from build123d import *

# Parameters (mm, degrees)
F4_DEPTH        = 101.6027760721
F5_R            = 1.5875
F6_DEPTH        = 127
F6_COPIES_COUNT = 5


# Not quite as in the source:
# - a pattern or mirror of a feature is missing from the dataset's text; its kind, count and spacing are read off the source's solid


with BuildPart() as f2:
    # F1 (on Front) → F2 (revolve)
    with BuildSketch(Plane.XZ):
        Polygon((-161.925, 101.2154587421), (-165.1, 101.2154587421), (-165.1, -0.3845412579), (-165.1, -6.7345412579), (0, -6.7345412579), (0, 0), (0, 228.6), (-6.35, 228.6), (-6.35, -0.3873173299), (-161.925, -0.3873173299), align=None)
    revolve(axis=Axis((0, 0, 5.5167637765), (0, 0, -1)))

    # F3 (on face) → F4 (cut, through all)
    with BuildSketch(Plane.XY.offset(101.2154587421)):
        with BuildLine():
            ThreePointArc((96.6025192728, -129.9525255435), (0, -161.925), (-96.6025192728, -129.9525255435))
            Line((-96.6025192728, -129.9525255435), (-96.6025192728, -133.8878757399))
            ThreePointArc((-96.6025192728, -133.8878757399), (0, -165.1), (96.6025192728, -133.8878757399))
            Line((96.6025192728, -133.8878757399), (96.6025192728, -129.9525255435))
        make_face()
    extrude(amount=-F4_DEPTH, mode=Mode.SUBTRACT)

    # F5 (on face) → F6 (join)
    with BuildSketch(Plane.XY.offset(101.2154587421)):
        with Locations((0, 163.5125)):
            Circle(F5_R)
    f6 = extrude(amount=F6_DEPTH)

    # F6_copies: F6 ×5 about axis
    f6_copies_axis = Axis((0, 0, 0), (0, 0, 1))
    for i in range(1, F6_COPIES_COUNT):
        add(f6.rotate(f6_copies_axis, i * 360 / F6_COPIES_COUNT))


solid = f2.part
Could you check a few things on this model? Use its own coordinates, in mm. A direction names the side the tool comes from. Round coordinates to 2 decimals unless told otherwise and drop trailing zeros. Write each loop counter-clockwise with the first axis right and the second up, starting at its lowest first coordinate (ties: lowest second). Pieces come first, ordered by that corner, then holes. Notation, with made-up numbers: (85.25, -7.5) - (111.25, -7.5) arc R25 cw to (111.25, 18.5) - close; hole circle Ø10 at (10, 85.5). An arc over 180 degrees is marked (long way). Use a Markdown table: item, result.
Q1. Please list where these lines run through material, in increasing order: L1, parallel to Y at x = 0, z = 73.5 (3 decimals); L2, parallel to Z at x = -38, y = 113.5; L3, parallel to X at y = 118, z = 85.5.
Output values:
| item | result |
|---|---|
| L1 | -6.35 to 6.35, 161.925 to 165.1 |
| L2 | -6.73 to -0.39 |
| L3 | -115.47 to -110.89, 110.89 to 115.47 |
Q2. For faces 1 (the flat face through (0, 0, 228.6)), 2 (the cylindrical face through (-5.672, 161.826, 51.125)), which set-ups out of +Z, -Z, +X, -X, +Y, -Y let a thin tool reach every point of the face, with its end or its side?
Output values:
| item | result |
|---|---|
| face 1 | +Z, +X, -X, +Y, -Y |
| face 2 | +Z |
Q3. I want a section at C-C (x = -56). List the corners of the cut face in (y, z) for me, plus the area to 3 significant figures.
Output values:
| item | result |
|---|---|
| outline | (-155.31, -6.73) - (155.31, -6.73) - (155.31, 101.22) - (151.93, 101.22) - (151.93, -0.39) - (-155.31, -0.39) - close |
| area | 2,310 mm2 |
Q4. I want a section at A-A (z = 32.5). List the corners of the cut face in (x, y) for me (3 decimals).
Output values:
| item | result |
|---|---|
| outline | (-96.603, -133.888) - (-96.603, -129.953) arc R161.925 cw (long way) to (96.603, -129.953) - (96.603, -133.888) arc R165.1 ccw (long way) to start; circle Ø12.7 at (0, 0) |
Q5. I want a section at B-B (y = 0). List the corners of the cut face in (x, z) for me (3 decimals), plus the area to 3 significant figures.
Output values:
| item | result |
|---|---|
| outline | (-165.1, -6.735) - (165.1, -6.735) - (165.1, 101.215) - (161.925, 101.215) - (161.925, -0.387) - (6.35, -0.387) - (6.35, 228.6) - (-6.35, 228.6) - (-6.35, -0.387) - (-161.925, -0.387) - (-161.925, 101.215) - (-165.1, 101.215) - close |
| area | 5,650 mm2 |
Q6. I want a section at D-D (z = 171.5). Count the separate pieces of the cut face and the enclosed holes in it, plus the area to 3 significant figures.
Output values:
| item | result |
|---|---|
| separate pieces | 6 |
| enclosed holes | 0 |
| area | 166 mm2 |
Q7. Thinking about a two-plate mould opening in X: for faces 3 (the flat face through (2, 2, -6.735)), 4 (the cylindrical face through (21.493, 163.695, 46.485)), 5 (the cylindrical face through (1.38, -6.2, 112.5)), which applies, released by +X, released by -X, zero draft, split by the parting line, or undercut?
Output values:
| item | result |
|---|---|
| face 3 | zero draft |
| face 4 | split by the parting line |
| face 5 | undercut |
Q8. For pin 1 (4 mm diameter, centred on x = 102.5, z = 55.5, fed in from +Y); pin 2 (3 mm diameter, centred on y = -132.5, z = 40, fed in from -X); pin 3 (4 mm diameter, centred on y = 118, z = 68, fed in from -X), each with a flat end and sliding along its axis, tell me the tip position at first contact or that it passes through.
Output values:
| item | result |
|---|---|
| pin 1 | y = 130.99 |
| pin 2 | x = -100.48 |
| pin 3 | x = -117.48 |
